```python
from build123d import *

# Parameters (mm, degrees)
BOSS_EXTRUDE1_DEPTH = 20
SHELL1_T            = -3
CUT_EXTRUDE1_DEPTH  = 40


with BuildPart() as part:
    # Sketch1 → Boss-Extrude1 (new, symmetric)
    with BuildSketch(Plane.XY):
        Polygon((40, 0), (0, 0), (0, 40), (5, 40), (40, 5), align=None)
    extrude(amount=BOSS_EXTRUDE1_DEPTH, both=True)

    # Shell1
    shell1_openings = [part.faces().sort_by_distance(p)[0] for p in [
        (22.5, 22.5, 0),
        (40, 2.5, 0),
        (2.5, 40, 0),
    ]]
    offset(amount=SHELL1_T, openings=shell1_openings, kind=Kind.INTERSECTION)

    # Sketch2 → Cut-Extrude1 (cut)
    with BuildSketch(Plane(origin=(3, 0, 0), x_dir=(0, 0, -1), z_dir=(1, 0, 0))):
        with BuildLine():
            Line((5, 27.5), (5, 17.5))
            ThreePointArc((5, 17.5), (0, 12.5), (-5, 17.5))
            Line((-5, 17.5), (-5, 27.5))
            ThreePointArc((-5, 27.5), (0, 32.5), (5, 27.5))
        make_face()
    cut_extrude1 = extrude(amount=-CUT_EXTRUDE1_DEPTH, mode=Mode.SUBTRACT)

    # Mirror1: Cut-Extrude1 across plane
    add(cut_extrude1.mirror(Plane(origin=(0, 0, 0), x_dir=(0, 0, 1), z_dir=(0.7071067811865476, -0.7071067811865476, 0))), mode=Mode.SUBTRACT)


solid = part.part
```
Can you work these out from the model? Positions are in its coordinate system, mm. A direction names the side the tool comes from. Round coordinates to 2 decimals unless told otherwise and drop trailing zeros. Loops run counter-clockwise (first coordinate to the right, second up) from the corner with the lowest first, then second, coordinate; pieces in that order, holes last. Notation, with made-up numbers: M 38,32 L 76,32 A22 cw 76,42 Z; hole C 18,-38 d10. An arc over 180 degrees is marked long. Answer in a Markdown table with one row per item.
1. If we section it at C-C, the plane y = 10.5: Please give me the cut outline in (x, z).
Established:
| item | result |
|---|---|
| outline | M 0,-20 L 34.5,-20 L 34.5,-17 L 3,-17 L 3,17 L 34.5,17 L 34.5,20 L 0,20 Z |
2. I'm going to push flat-ended pins straight in: pin 1 Ø17 at (x, z) = (21.5, -6.5) entering from +Y; pin 2 Ø3 at (y, z) = (27, 14) entering from -X; pin 3 Ø12 at (y, z) = (17, -2) entering from +X; pin 4 Ø1.5 at (y, z) = (26.5, -3) entering from +X. Where does each tip first touch, or does it pass through?
Established:
| item | result |
|---|---|
| pin 1 | y = 3 |
| pin 2 | x = 0 |
| pin 3 | x = 3 |
| pin 4 | through |
3. Please list where these lines run through material, in increasing order: line 1 (Z direction, x = 21, y = 5); line 2 (X direction, y = 21, z = 6.5). Write a range as from..to.
Established:
| item | result |
|---|---|
| line 1 | -20..-17, 17..20 |
| line 2 | 0..3 |
4. On a 3-axis mill with a long thin cutter (end or side, diameter ignored), from which of +Z, -Z, +X, -X, +Y, -Y can I reach the whole of each face in a straight line? I mean faces 5 (the face through (3, 21, -7)), 6 (the face through (40, 2, 0)), 7 (the face through (2, 22, 5)), 8 (the face through (22, 2, 5)), 9 (the face through (16, 0, 5)). Say none if no direction works.
Established:
| item | result |
|---|---|
| face 5 | +X, +Y |
| face 6 | +Z, -Z, +X, +Y, -Y |
| face 7 | +X, -X |
| face 8 | +Y, -Y |
| face 9 | +Z, -Z, +X, -X, -Y |
5. If we section it at B-B, the plane z = 0: Please give me the cut outline in (x, y).
Established:
| item | result |
|---|---|
| outline | M 0,0 L 12.5,0 L 12.5,3 L 3,3 L 3,12.5 L 0,12.5 Z; M 0,32.5 L 3,32.5 L 3,40 L 0,40 Z; M 32.5,0 L 40,0 L 40,3 L 32.5,3 Z |
6. If we section it at A-A, the plane y = 20.5: Please give me the cut outline in (x, z), plus the area to 3 significant figures.
Established:
| item | result |
|---|---|
| outline | M 0,-20 L 24.5,-20 L 24.5,-17 L 3,-17 L 3,-5 L 0,-5 Z; M 0,5 L 3,5 L 3,17 L 24.5,17 L 24.5,20 L 0,20 Z |
| area | 219 mm² |
7. If we section it at D-D, the plane x = 33.5: Please give me the cut outline in (y, z).
Established:
| item | result |
|---|---|
| outline | M 0,-20 L 11.5,-20 L 11.5,-17 L 3,-17 L 3,17 L 11.5,17 L 11.5,20 L 0,20 Z |
8. Thinking about a two-plate mould opening in Y: for faces 1 (the face through (22, 23, 19)), 2 (the face through (2, 23, -5)), 3 (the face through (16, 16, -20)), 4 (the face through (1.5, 32.5, 0.1)), which applies, pulls with the +Y half, pulls with the -Y half, needs draft (parallel to the pull), parting line crosses it, or undercut?
Established:
| item | result |
|---|---|
| face 1 | pulls with the +Y half |
| face 2 | undercut |
| face 3 | needs draft |
| face 4 | undercut |
